from build123d import *

# Parameters (mm, degrees)
F0_W      = 12
F0_H      = 12
F1_DEPTH  = 6
F2_R      = 1.25
F3_DEPTH  = 12.001
F4_R      = 1.25
F5_DEPTH  = 3
F6_R      = 1.25
F7_DEPTH  = 25
F8_R      = 2
F9_W      = 1
F9_H      = 1
F10_DEPTH = 3


with BuildPart() as f1:
    # F0 (on Right) → F1 (new body, symmetric)
    with BuildSketch(Plane.YZ):
        Rectangle(F0_W, F0_H)
    extrude(amount=F1_DEPTH, both=True)

    # F2 (on face) → F3 (cut, through all)
    with BuildSketch(Plane.YZ.offset(6)):
        Circle(F2_R)
    extrude(amount=-F3_DEPTH, mode=Mode.SUBTRACT)

    # F4 (on face) → F5 (cut)
    with BuildSketch(Plane(origin=(0, 6, 0), x_dir=(-1, 0, 0), z_dir=(0, 1, 0))):
        Circle(F4_R)
    extrude(amount=-F5_DEPTH, mode=Mode.SUBTRACT)

    # F6 (on face) → F7 (cut)
    with BuildSketch(Plane(origin=(0, 0, -6), x_dir=(1, 0, 0), z_dir=(0, 0, -1))):
        Circle(F6_R)
    extrude(amount=-F7_DEPTH, mode=Mode.SUBTRACT)

    # F8
    f8_edges = [f1.edges().sort_by_distance(p)[0] for p in [
        (6, 6, 0),
        (-6, 6, 0),
        (-6, 0, -6),
        (6, 0, -6),
        (0, 6, -6),
        (-6, 0, 6),
        (0, 6, 6),
        (6, 0, 6),
    ]]
    fillet(f8_edges, radius=F8_R)

    # F9 (on face) → F10 (cut)
    with BuildSketch(Plane.XZ.offset(6)):
        with Locations((-4, 4)):
            Rectangle(F9_W, F9_H)
        with Locations((-4, 2.4)):
            Rectangle(F9_W, F9_H)
        with Locations((-4, 0.8)):
            Rectangle(F9_W, F9_H)
        with Locations((-4, -0.8)):
            Rectangle(F9_W, F9_H)
        with Locations((-4, -2.4)):
            Rectangle(F9_W, F9_H)
        with Locations((-4, -4)):
            Rectangle(F9_W, F9_H)
        with Locations((-2.4, 4)):
            Rectangle(F9_W, F9_H)
        with Locations((-2.4, 2.4)):
            Rectangle(F9_W, F9_H)
        with Locations((-2.4, 0.8)):
            Rectangle(F9_W, F9_H)
        with Locations((-2.4, -0.8)):
            Rectangle(F9_W, F9_H)
        with Locations((-2.4, -2.4)):
            Rectangle(F9_W, F9_H)
        with Locations((-2.4, -4)):
            Rectangle(F9_W, F9_H)
        with Locations((-0.8, 4)):
            Rectangle(F9_W, F9_H)
        with Locations((-0.8, 2.4)):
            Rectangle(F9_W, F9_H)
        with Locations((-0.8, 0.8)):
            Rectangle(F9_W, F9_H)
        with Locations((-0.8, -0.8)):
            Rectangle(F9_W, F9_H)
        with Locations((-0.8, -2.4)):
            Rectangle(F9_W, F9_H)
        with Locations((-0.8, -4)):
            Rectangle(F9_W, F9_H)
        with Locations((0.8, 4)):
            Rectangle(F9_W, F9_H)
        with Locations((0.8, 2.4)):
            Rectangle(F9_W, F9_H)
        with Locations((0.8, 0.8)):
            Rectangle(F9_W, F9_H)
        with Locations((0.8, -0.8)):
            Rectangle(F9_W, F9_H)
        with Locations((0.8, -2.4)):
            Rectangle(F9_W, F9_H)
        with Locations((0.8, -4)):
            Rectangle(F9_W, F9_H)
        with Locations((2.4, 4)):
            Rectangle(F9_W, F9_H)
        with Locations((2.4, 2.4)):
            Rectangle(F9_W, F9_H)
        with Locations((2.4, 0.8)):
            Rectangle(F9_W, F9_H)
        with Locations((2.4, -0.8)):
            Rectangle(F9_W, F9_H)
        with Locations((2.4, -2.4)):
            Rectangle(F9_W, F9_H)
        with Locations((2.4, -4)):
            Rectangle(F9_W, F9_H)
        with Locations((4, 4)):
            Rectangle(F9_W, F9_H)
        with Locations((4, 2.4)):
            Rectangle(F9_W, F9_H)
        with Locations((4, 0.8)):
            Rectangle(F9_W, F9_H)
        with Locations((4, -0.8)):
            Rectangle(F9_W, F9_H)
        with Locations((4, -2.4)):
            Rectangle(F9_W, F9_H)
        with Locations((4, -4)):
            Rectangle(F9_W, F9_H)
    extrude(amount=-F10_DEPTH, mode=Mode.SUBTRACT)


solid = f1.part
Verification items for the finished model (mm, model axes). A direction names the side the tool comes from. Give positions to 0.01 mm unless a question says otherwise; leave off trailing zeros. Write each loop counter-clockwise with the first axis right and the second up, starting at its lowest first coordinate (ties: lowest second). Pieces come first, ordered by that corner, then holes. Notation, with made-up numbers: (-23, 82.5) - (-4, 82.5) arc R7 cw to (-4, 91.5) - close; hole circle Ø3 at (79, 74). An arc over 180 degrees is marked (long way). Answer as CSV lines item,"result". Start each with the question number.
1. Set-up check for faces 1 (the face through (1, -1, 6)), 2 (the face through (2.9, -4.5, -2.4)): record each of +Z, -Z, +X, -X, +Y, -Y from which the full face is reachable in a straight line by a thin tool's end or side.
2. Draft check along X on faces 3 (the face through (-4, -3, -2.4)), 4 (the face through (0.06, 5.4, -5.43)). Enter one of: pulls with the +X half, pulls with the -X half, needs draft (parallel to the pull), parting line crosses it, or undercut.
3. Sectioned sample at C-C (y = 0). Record the boundary of the cut face in (x, z).
4. Sectioned sample at A-A (y = 3.5). Record the boundary of the cut face in (x, z), then the cut area to 3 significant figures.
5. Thickness scan on line 1 (Z direction, x = -3.9, y = 0); line 2 (Y direction, x = 4, z = -2.5). Record the ranges inside material, lowest first.
6. Sectioned sample at D-D (y = -4.5). Count the separate pieces of the cut face and the enclosed holes in it, then the cut area to 3 significant figures.
Derived:
1,face 1,"+Z, +X, -X, +Y, -Y"
1,face 2,"-Y"
2,face 3,"undercut"
2,face 4,"needs draft"
3,outline,"(-6, -4) arc R2 ccw to (-4, -6) - (-1.25, -6) - (-1.25, -1.25) - (-6, -1.25) - close; (-6, 1.25) - (-1.25, 1.25) - (-1.25, 6) - (-4, 6) arc R2 ccw to (-6, 4) - close; (1.25, -6) - (4, -6) arc R2 ccw to (6, -4) - (6, -1.25) - (1.25, -1.25) - close; (1.25, 1.25) - (6, 1.25) - (6, 4) arc R2 ccw to (4, 6) - (1.25, 6) - close"
4,outline,"(-6, -4) arc R2 ccw to (-4, -6) - (4, -6) arc R2 ccw to (6, -4) - (6, 4) arc R2 ccw to (4, 6) - (-4, 6) arc R2 ccw to (-6, 4) - close; hole circle Ø2.5 at (0, 0)"
4,area,"136 mm²"
5,line 1,"-6 to -1.25, 1.25 to 6"
5,line 2,"-3 to 6"
6,separate pieces,"1"
6,enclosed holes,"36"
6,area,"105 mm²"
